Could you check a few things on this model? Use its own coordinates, in mm. Round coordinates to 2 decimals unless told otherwise and drop trailing zeros. Loops run counter-clockwise (first coordinate to the right, second up) from the corner with the lowest first, then second, coordinate; pieces in that order, holes last. Notation, with made-up numbers: (-25.5, -25.5) - (3.5, -25.5) arc R19 cw to (3.5, -14.5) - close; hole circle Ø2 at (-24.5, 83). An arc over 180 degrees is marked (long way). Put each result on its own line as item: value. Start each with the question number.
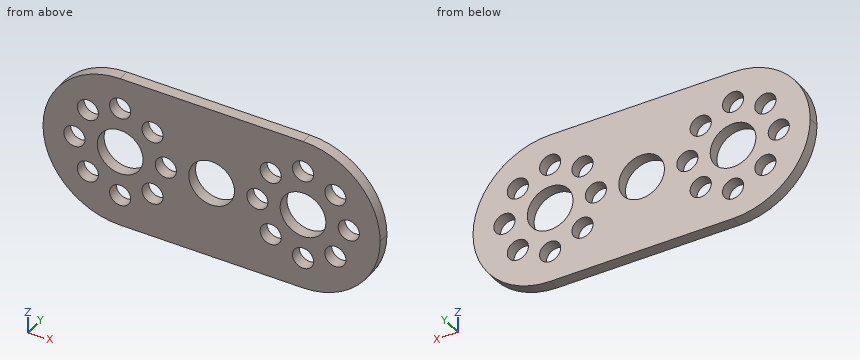
from build123d import *

# Parameters (mm, degrees)
F0_R     = 1.85
F0_R_2   = 4
F1_DEPTH = 2


with BuildPart() as f1:
    # F0 (on Front) → F1 (new body)
    with BuildSketch(Plane.XZ):
        with BuildLine():
            ThreePointArc((29.5, 0), (25.545942, 9.545942), (16, 13.5))
            Line((16, 13.5), (-16, 13.5))
            ThreePointArc((-16, 13.5), (-25.545942, 9.545942), (-29.5, 0))
            ThreePointArc((-29.5, 0), (-25.545942, -9.545942), (-16, -13.5))
            Line((-16, -13.5), (16, -13.5))
            ThreePointArc((16, -13.5), (25.545942, -9.545942), (29.5, 0))
        make_face()
        with Locations((-16, -8)):
            Circle(F0_R, mode=Mode.SUBTRACT)
        with Locations((-21.656854, -5.656854)):
            Circle(F0_R, mode=Mode.SUBTRACT)
        with Locations((-10.343146, -5.656854)):
            Circle(F0_R, mode=Mode.SUBTRACT)
        with Locations((16, -8)):
            Circle(F0_R, mode=Mode.SUBTRACT)
        with Locations((10.343146, -5.656854)):
            Circle(F0_R, mode=Mode.SUBTRACT)
        with Locations((21.656854, -5.656854)):
            Circle(F0_R, mode=Mode.SUBTRACT)
        with Locations((-24, 0)):
            Circle(F0_R, mode=Mode.SUBTRACT)
        with Locations((-16, 0)):
            Circle(F0_R_2, mode=Mode.SUBTRACT)
        with Locations((-21.656854, 5.656854)):
            Circle(F0_R, mode=Mode.SUBTRACT)
        with Locations((-8, 0)):
            Circle(F0_R, mode=Mode.SUBTRACT)
        with Locations((-10.343146, 5.656854)):
            Circle(F0_R, mode=Mode.SUBTRACT)
        with Locations((-16, 8)):
            Circle(F0_R, mode=Mode.SUBTRACT)
        Circle(F0_R_2, mode=Mode.SUBTRACT)
        with Locations((8, 0)):
            Circle(F0_R, mode=Mode.SUBTRACT)
        with Locations((10.343146, 5.656854)):
            Circle(F0_R, mode=Mode.SUBTRACT)
        with Locations((16, 0)):
            Circle(F0_R_2, mode=Mode.SUBTRACT)
        with Locations((24, 0)):
            Circle(F0_R, mode=Mode.SUBTRACT)
        with Locations((21.656854, 5.656854)):
            Circle(F0_R, mode=Mode.SUBTRACT)
        with Locations((16, 8)):
            Circle(F0_R, mode=Mode.SUBTRACT)
    extrude(amount=F1_DEPTH)


solid = f1.part
Item 1: Suppose I cut it at C-C, the plane y = -1.45. Count the separate pieces of the cut face and the enclosed holes in it, then the cut area to 3 significant figures.
Item 2: Suppose I cut it at D-D, the plane z = 6.75. List the corners of the cut face in (x, y) for me.
Item 3: Suppose I cut it at B-B, the plane x = 3. List the corners of the cut face in (y, z) for me, then the cut area to 3 significant figures.
Item 4: Will this pin go through, and if not, where does the flat tip stop? P1, Ø2, axis at x = -21.66, z = 5.66, coming from the +Y side.
Item 5: I need wall thicknesses on line 1 (Z direction, x = 16, y = -1.4); line 2 (X direction, y = -0.5, z = 9); line 3 (Z direction, x = -21.5, y = -1.15). Which ranges of each line are inside material? Lowest first, please. Write a range as from..to.
Item 6: Suppose I cut it at A-A, the plane z = -4.75. List the corners of the cut face in (x, y) for me.
Numbers:
1. separate pieces: 1
1. enclosed holes: 19
1. area: 1,110 mm^2
2. outline: (-27.69, -2) - (-23.15, -2) - (-23.15, 0) - (-27.69, 0) - close; (-20.16, -2) - (-17.36, -2) - (-17.36, 0) - (-20.16, 0) - close; (-14.64, -2) - (-11.84, -2) - (-11.84, 0) - (-14.64, 0) - close; (-8.85, -2) - (8.85, -2) - (8.85, 0) - (-8.85, 0) - close; (11.84, -2) - (14.64, -2) - (14.64, 0) - (11.84, 0) - close; (17.36, -2) - (20.16, -2) - (20.16, 0) - (17.36, 0) - close; (23.15, -2) - (27.69, -2) - (27.69, 0) - (23.15, 0) - close
3. outline: (-2, -13.5) - (0, -13.5) - (0, -2.65) - (-2, -2.65) - close; (-2, 2.65) - (0, 2.65) - (0, 13.5) - (-2, 13.5) - close
3. area: 43.4 mm^2
4. P1: through
5. line 1: -13.5..-9.85, -6.15..-4, 4..6.15, 9.85..13.5
5. line 2: -26.06..-17.56, -14.44..14.44, 17.56..26.06
5. line 3: -12.33..-7.5, -3.81..3.81, 7.5..12.33
6. outline: (-28.64, -2) - (-23.27, -2) - (-23.27, 0) - (-28.64, 0) - close; (-20.04, -2) - (-11.96, -2) - (-11.96, 0) - (-20.04, 0) - close; (-8.73, -2) - (8.73, -2) - (8.73, 0) - (-8.73, 0) - close; (11.96, -2) - (20.04, -2) - (20.04, 0) - (11.96, 0) - close; (23.27, -2) - (28.64, -2) - (28.64, 0) - (23.27, 0) - close
